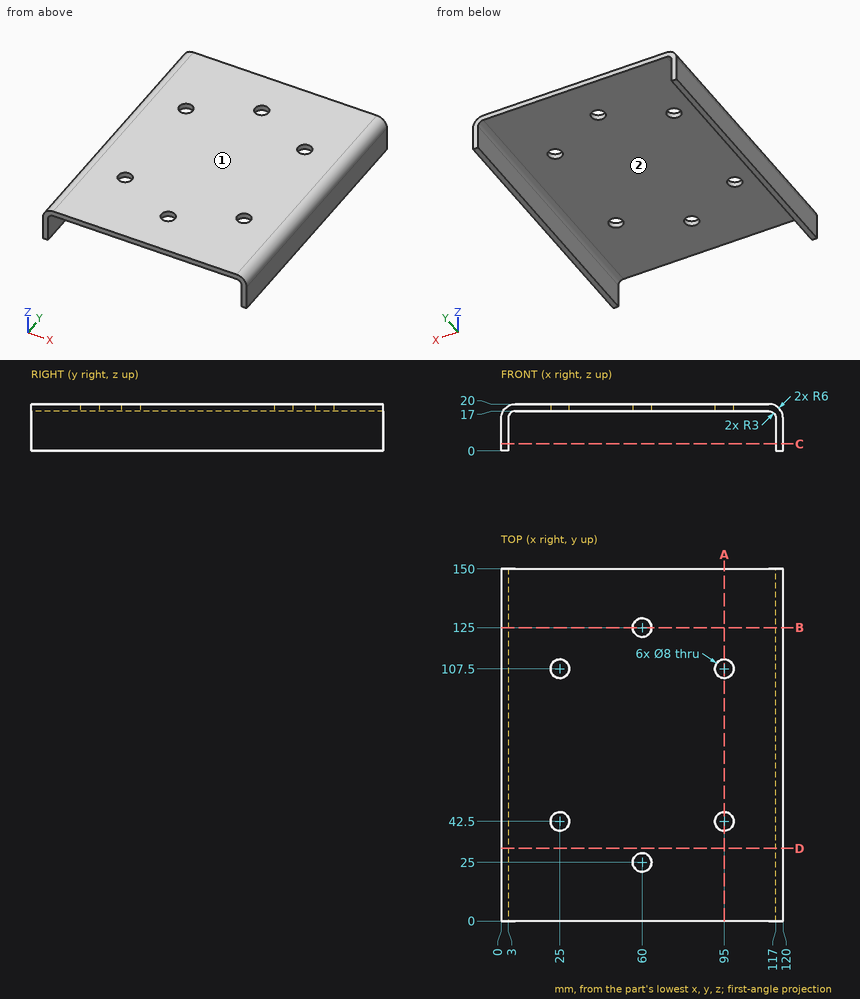
Geometry check sheet. Reference: drawing and pictorial views, mm from the part's lowest x, y, z. Round coordinates to 2 decimals unless told otherwise and drop trailing zeros. Write each loop counter-clockwise with the first axis right and the second up, starting at its lowest first coordinate (ties: lowest second). Pieces come first, ordered by that corner, then holes.
1. Draft check along X on the marked faces 1 and 2. Enter one of: +X half, -X half, draft (parallel to the pull), parting line (faces both ways), or undercut.
2. Gauge pin test, flat end, axial feed: P1, Ø13, axis at x = 95, y = 42.5, coming from the -Z side. Record the tip position at first contact, or that the pin passes through.
3. Section check A-A on x = 95. Enter the section's corners in (y, z).
4. Section check D-D on y = 31. Enter the section's corners in (x, z), plus the area to 3 significant figures.
5. Section check B-B on y = 125. Enter the section's corners in (x, z), plus the area to 3 significant figures.
6. Section check C-C on z = 3. Enter the section's corners in (x, y).
7. Scan lines: L1, parallel to Y at x = 25, z = 18.9; L2, parallel to Y at x = 60, z = 18.25; L3, parallel to X at y = 7, z = 14.25. Record each from-to range of solid material in increasing order.
Answer:
1. face 1: draft
1. face 2: undercut
2. P1: stops at z = 17
3. outline: (0, 17) - (38.5, 17) - (38.5, 20) - (0, 20) - close; (46.5, 17) - (103.5, 17) - (103.5, 20) - (46.5, 20) - close; (111.5, 17) - (150, 17) - (150, 20) - (111.5, 20) - close
4. outline: (0, 0) - (3, 0) - (3, 14) arc R3 cw to (6, 17) - (114, 17) arc R3 cw to (117, 14) - (117, 0) - (120, 0) - (120, 14) arc R6 ccw to (114, 20) - (6, 20) arc R6 ccw to (0, 14) - close
4. area: 450 mm2
5. outline: (0, 0) - (3, 0) - (3, 14) arc R3 cw to (6, 17) - (56, 17) - (56, 20) - (6, 20) arc R6 ccw to (0, 14) - close; (64, 17) - (114, 17) arc R3 cw to (117, 14) - (117, 0) - (120, 0) - (120, 14) arc R6 ccw to (114, 20) - (64, 20) - close
5. area: 426 mm2
6. outline: (0, 0) - (3, 0) - (3, 150) - (0, 150) - close; (117, 0) - (120, 0) - (120, 150) - (117, 150) - close
7. L1: y = 0 to 38.5, 46.5 to 103.5, 111.5 to 150
7. L2: y = 0 to 21, 29 to 121, 129 to 150
7. L3: x = 0.01 to 3.01, 116.99 to 119.99
